Verification items for the finished model (mm, model axes). A direction names the side the tool comes from. Round coordinates to 2 decimals unless told otherwise and drop trailing zeros. Loops run counter-clockwise (first coordinate to the right, second up) from the corner with the lowest first, then second, coordinate; pieces in that order, holes last. Notation, with made-up numbers: M 42,67 L 83,67 A20 cw 83,85 Z; hole C 11,82.25 d10. An arc over 180 degrees is marked long. Write item = value, one per line. Start each with the question number.
from build123d import *

# Parameters (mm, degrees)
SKETCH1_W                  = 30
SKETCH1_H                  = 330
BOSS_EXTRUDE1_DEPTH        = 8.4
SKETCH2_R                  = 1
CUT_EXTRUDE1_DEPTH         = 332.467283453
LPATTERN1_COUNT            = 30
LPATTERN1_PITCH            = 8.5
LPATTERN2_COUNT            = 2
LPATTERN2_PITCH            = 22
LPATTERN2_COPY_1_SKETCH_R  = 1
LPATTERN2_COPY_1_DEPTH     = 332.467283453
LPATTERN2_COPY_2_SKETCH_R  = 1
LPATTERN2_COPY_2_DEPTH     = 332.467283453
LPATTERN2_COPY_3_SKETCH_R  = 1
LPATTERN2_COPY_3_DEPTH     = 332.467283453
LPATTERN2_COPY_4_SKETCH_R  = 1
LPATTERN2_COPY_4_DEPTH     = 332.467283453
LPATTERN2_COPY_5_SKETCH_R  = 1
LPATTERN2_COPY_5_DEPTH     = 332.467283453
LPATTERN2_COPY_6_SKETCH_R  = 1
LPATTERN2_COPY_6_DEPTH     = 332.467283453
LPATTERN2_COPY_7_SKETCH_R  = 1
LPATTERN2_COPY_7_DEPTH     = 332.467283453
LPATTERN2_COPY_8_SKETCH_R  = 1
LPATTERN2_COPY_8_DEPTH     = 332.467283453
LPATTERN2_COPY_9_SKETCH_R  = 1
LPATTERN2_COPY_9_DEPTH     = 332.467283453
LPATTERN2_COPY_10_SKETCH_R = 1
LPATTERN2_COPY_10_DEPTH    = 332.467283453
LPATTERN2_COPY_11_SKETCH_R = 1
LPATTERN2_COPY_11_DEPTH    = 332.467283453
LPATTERN2_COPY_12_SKETCH_R = 1
LPATTERN2_COPY_12_DEPTH    = 332.467283453
LPATTERN2_COPY_13_SKETCH_R = 1
LPATTERN2_COPY_13_DEPTH    = 332.467283453
LPATTERN2_COPY_14_SKETCH_R = 1
LPATTERN2_COPY_14_DEPTH    = 332.467283453
LPATTERN2_COPY_15_SKETCH_R = 1
LPATTERN2_COPY_15_DEPTH    = 332.467283453
LPATTERN2_COPY_16_SKETCH_R = 1
LPATTERN2_COPY_16_DEPTH    = 332.467283453
LPATTERN2_COPY_17_SKETCH_R = 1
LPATTERN2_COPY_17_DEPTH    = 332.467283453
LPATTERN2_COPY_18_SKETCH_R = 1
LPATTERN2_COPY_18_DEPTH    = 332.467283453
LPATTERN2_COPY_19_SKETCH_R = 1
LPATTERN2_COPY_19_DEPTH    = 332.467283453
LPATTERN2_COPY_20_SKETCH_R = 1
LPATTERN2_COPY_20_DEPTH    = 332.467283453
LPATTERN2_COPY_21_SKETCH_R = 1
LPATTERN2_COPY_21_DEPTH    = 332.467283453
LPATTERN2_COPY_22_SKETCH_R = 1
LPATTERN2_COPY_22_DEPTH    = 332.467283453
LPATTERN2_COPY_23_SKETCH_R = 1
LPATTERN2_COPY_23_DEPTH    = 332.467283453
LPATTERN2_COPY_24_SKETCH_R = 1
LPATTERN2_COPY_24_DEPTH    = 332.467283453
LPATTERN2_COPY_25_SKETCH_R = 1
LPATTERN2_COPY_25_DEPTH    = 332.467283453
LPATTERN2_COPY_26_SKETCH_R = 1
LPATTERN2_COPY_26_DEPTH    = 332.467283453
LPATTERN2_COPY_27_SKETCH_R = 1
LPATTERN2_COPY_27_DEPTH    = 332.467283453
LPATTERN2_COPY_28_SKETCH_R = 1
LPATTERN2_COPY_28_DEPTH    = 332.467283453
LPATTERN2_COPY_29_SKETCH_R = 1
LPATTERN2_COPY_29_DEPTH    = 332.467283453
SKETCH4_W                  = 24
SKETCH4_H                  = 65
CUT_EXTRUDE2_DEPTH         = 1.6
SKETCH6_W                  = 24
SKETCH6_H                  = 10
CUT_EXTRUDE3_DEPTH         = 1.6
SKETCH7_W                  = 30
SKETCH7_H                  = 8.4
BOSS_EXTRUDE2_DEPTH        = 2
SKETCH8_R                  = 2.5
CUT_EXTRUDE4_DEPTH         = 334.458483173


with BuildPart() as part:
    # Sketch1 → Boss-Extrude1 (new body)
    with BuildSketch(Plane.XY):
        with Locations((15, 165)):
            Rectangle(SKETCH1_W, SKETCH1_H)
    extrude(amount=BOSS_EXTRUDE1_DEPTH)

    # Sketch2 → Cut-Extrude1 (cut, through all)
    with BuildSketch(Plane.XY.offset(8.4)):
        with Locations((26, 4)):
            Circle(SKETCH2_R)
    cut_extrude1 = extrude(amount=-CUT_EXTRUDE1_DEPTH, mode=Mode.SUBTRACT)

    # LPattern1: Cut-Extrude1 ×30
    with Locations(*[(0, i * LPATTERN1_PITCH, 0) for i in range(1, LPATTERN1_COUNT)]):
        add(cut_extrude1, mode=Mode.SUBTRACT)

    # LPattern2: Cut-Extrude1 ×2
    with Locations(*[(-i * LPATTERN2_PITCH, 0, 0) for i in range(1, LPATTERN2_COUNT)]):
        add(cut_extrude1, mode=Mode.SUBTRACT)

    # LPattern2 copy 1 sketch → LPattern2 copy 1 (cut, through all)
    with BuildSketch(Plane(origin=(-22, 8.5, 8.4), x_dir=(1, 0, 0), z_dir=(0, 0, 1))):
        with Locations((26, 4)):
            Circle(LPATTERN2_COPY_1_SKETCH_R)
    extrude(amount=-LPATTERN2_COPY_1_DEPTH, mode=Mode.SUBTRACT)

    # LPattern2 copy 2 sketch → LPattern2 copy 2 (cut, through all)
    with BuildSketch(Plane(origin=(-22, 17, 8.4), x_dir=(1, 0, 0), z_dir=(0, 0, 1))):
        with Locations((26, 4)):
            Circle(LPATTERN2_COPY_2_SKETCH_R)
    extrude(amount=-LPATTERN2_COPY_2_DEPTH, mode=Mode.SUBTRACT)

    # LPattern2 copy 3 sketch → LPattern2 copy 3 (cut, through all)
    with BuildSketch(Plane(origin=(-22, 25.5, 8.4), x_dir=(1, 0, 0), z_dir=(0, 0, 1))):
        with Locations((26, 4)):
            Circle(LPATTERN2_COPY_3_SKETCH_R)
    extrude(amount=-LPATTERN2_COPY_3_DEPTH, mode=Mode.SUBTRACT)

    # LPattern2 copy 4 sketch → LPattern2 copy 4 (cut, through all)
    with BuildSketch(Plane(origin=(-22, 34, 8.4), x_dir=(1, 0, 0), z_dir=(0, 0, 1))):
        with Locations((26, 4)):
            Circle(LPATTERN2_COPY_4_SKETCH_R)
    extrude(amount=-LPATTERN2_COPY_4_DEPTH, mode=Mode.SUBTRACT)

    # LPattern2 copy 5 sketch → LPattern2 copy 5 (cut, through all)
    with BuildSketch(Plane(origin=(-22, 42.5, 8.4), x_dir=(1, 0, 0), z_dir=(0, 0, 1))):
        with Locations((26, 4)):
            Circle(LPATTERN2_COPY_5_SKETCH_R)
    extrude(amount=-LPATTERN2_COPY_5_DEPTH, mode=Mode.SUBTRACT)

    # LPattern2 copy 6 sketch → LPattern2 copy 6 (cut, through all)
    with BuildSketch(Plane(origin=(-22, 51, 8.4), x_dir=(1, 0, 0), z_dir=(0, 0, 1))):
        with Locations((26, 4)):
            Circle(LPATTERN2_COPY_6_SKETCH_R)
    extrude(amount=-LPATTERN2_COPY_6_DEPTH, mode=Mode.SUBTRACT)

    # LPattern2 copy 7 sketch → LPattern2 copy 7 (cut, through all)
    with BuildSketch(Plane(origin=(-22, 59.5, 8.4), x_dir=(1, 0, 0), z_dir=(0, 0, 1))):
        with Locations((26, 4)):
            Circle(LPATTERN2_COPY_7_SKETCH_R)
    extrude(amount=-LPATTERN2_COPY_7_DEPTH, mode=Mode.SUBTRACT)

    # LPattern2 copy 8 sketch → LPattern2 copy 8 (cut, through all)
    with BuildSketch(Plane(origin=(-22, 68, 8.4), x_dir=(1, 0, 0), z_dir=(0, 0, 1))):
        with Locations((26, 4)):
            Circle(LPATTERN2_COPY_8_SKETCH_R)
    extrude(amount=-LPATTERN2_COPY_8_DEPTH, mode=Mode.SUBTRACT)

    # LPattern2 copy 9 sketch → LPattern2 copy 9 (cut, through all)
    with BuildSketch(Plane(origin=(-22, 76.5, 8.4), x_dir=(1, 0, 0), z_dir=(0, 0, 1))):
        with Locations((26, 4)):
            Circle(LPATTERN2_COPY_9_SKETCH_R)
    extrude(amount=-LPATTERN2_COPY_9_DEPTH, mode=Mode.SUBTRACT)

    # LPattern2 copy 10 sketch → LPattern2 copy 10 (cut, through all)
    with BuildSketch(Plane(origin=(-22, 85, 8.4), x_dir=(1, 0, 0), z_dir=(0, 0, 1))):
        with Locations((26, 4)):
            Circle(LPATTERN2_COPY_10_SKETCH_R)
    extrude(amount=-LPATTERN2_COPY_10_DEPTH, mode=Mode.SUBTRACT)

    # LPattern2 copy 11 sketch → LPattern2 copy 11 (cut, through all)
    with BuildSketch(Plane(origin=(-22, 93.5, 8.4), x_dir=(1, 0, 0), z_dir=(0, 0, 1))):
        with Locations((26, 4)):
            Circle(LPATTERN2_COPY_11_SKETCH_R)
    extrude(amount=-LPATTERN2_COPY_11_DEPTH, mode=Mode.SUBTRACT)

    # LPattern2 copy 12 sketch → LPattern2 copy 12 (cut, through all)
    with BuildSketch(Plane(origin=(-22, 102, 8.4), x_dir=(1, 0, 0), z_dir=(0, 0, 1))):
        with Locations((26, 4)):
            Circle(LPATTERN2_COPY_12_SKETCH_R)
    extrude(amount=-LPATTERN2_COPY_12_DEPTH, mode=Mode.SUBTRACT)

    # LPattern2 copy 13 sketch → LPattern2 copy 13 (cut, through all)
    with BuildSketch(Plane(origin=(-22, 110.5, 8.4), x_dir=(1, 0, 0), z_dir=(0, 0, 1))):
        with Locations((26, 4)):
            Circle(LPATTERN2_COPY_13_SKETCH_R)
    extrude(amount=-LPATTERN2_COPY_13_DEPTH, mode=Mode.SUBTRACT)

    # LPattern2 copy 14 sketch → LPattern2 copy 14 (cut, through all)
    with BuildSketch(Plane(origin=(-22, 119, 8.4), x_dir=(1, 0, 0), z_dir=(0, 0, 1))):
        with Locations((26, 4)):
            Circle(LPATTERN2_COPY_14_SKETCH_R)
    extrude(amount=-LPATTERN2_COPY_14_DEPTH, mode=Mode.SUBTRACT)

    # LPattern2 copy 15 sketch → LPattern2 copy 15 (cut, through all)
    with BuildSketch(Plane(origin=(-22, 127.5, 8.4), x_dir=(1, 0, 0), z_dir=(0, 0, 1))):
        with Locations((26, 4)):
            Circle(LPATTERN2_COPY_15_SKETCH_R)
    extrude(amount=-LPATTERN2_COPY_15_DEPTH, mode=Mode.SUBTRACT)

    # LPattern2 copy 16 sketch → LPattern2 copy 16 (cut, through all)
    with BuildSketch(Plane(origin=(-22, 136, 8.4), x_dir=(1, 0, 0), z_dir=(0, 0, 1))):
        with Locations((26, 4)):
            Circle(LPATTERN2_COPY_16_SKETCH_R)
    extrude(amount=-LPATTERN2_COPY_16_DEPTH, mode=Mode.SUBTRACT)

    # LPattern2 copy 17 sketch → LPattern2 copy 17 (cut, through all)
    with BuildSketch(Plane(origin=(-22, 144.5, 8.4), x_dir=(1, 0, 0), z_dir=(0, 0, 1))):
        with Locations((26, 4)):
            Circle(LPATTERN2_COPY_17_SKETCH_R)
    extrude(amount=-LPATTERN2_COPY_17_DEPTH, mode=Mode.SUBTRACT)

    # LPattern2 copy 18 sketch → LPattern2 copy 18 (cut, through all)
    with BuildSketch(Plane(origin=(-22, 153, 8.4), x_dir=(1, 0, 0), z_dir=(0, 0, 1))):
        with Locations((26, 4)):
            Circle(LPATTERN2_COPY_18_SKETCH_R)
    extrude(amount=-LPATTERN2_COPY_18_DEPTH, mode=Mode.SUBTRACT)

    # LPattern2 copy 19 sketch → LPattern2 copy 19 (cut, through all)
    with BuildSketch(Plane(origin=(-22, 161.5, 8.4), x_dir=(1, 0, 0), z_dir=(0, 0, 1))):
        with Locations((26, 4)):
            Circle(LPATTERN2_COPY_19_SKETCH_R)
    extrude(amount=-LPATTERN2_COPY_19_DEPTH, mode=Mode.SUBTRACT)

    # LPattern2 copy 20 sketch → LPattern2 copy 20 (cut, through all)
    with BuildSketch(Plane(origin=(-22, 170, 8.4), x_dir=(1, 0, 0), z_dir=(0, 0, 1))):
        with Locations((26, 4)):
            Circle(LPATTERN2_COPY_20_SKETCH_R)
    extrude(amount=-LPATTERN2_COPY_20_DEPTH, mode=Mode.SUBTRACT)

    # LPattern2 copy 21 sketch → LPattern2 copy 21 (cut, through all)
    with BuildSketch(Plane(origin=(-22, 178.5, 8.4), x_dir=(1, 0, 0), z_dir=(0, 0, 1))):
        with Locations((26, 4)):
            Circle(LPATTERN2_COPY_21_SKETCH_R)
    extrude(amount=-LPATTERN2_COPY_21_DEPTH, mode=Mode.SUBTRACT)

    # LPattern2 copy 22 sketch → LPattern2 copy 22 (cut, through all)
    with BuildSketch(Plane(origin=(-22, 187, 8.4), x_dir=(1, 0, 0), z_dir=(0, 0, 1))):
        with Locations((26, 4)):
            Circle(LPATTERN2_COPY_22_SKETCH_R)
    extrude(amount=-LPATTERN2_COPY_22_DEPTH, mode=Mode.SUBTRACT)

    # LPattern2 copy 23 sketch → LPattern2 copy 23 (cut, through all)
    with BuildSketch(Plane(origin=(-22, 195.5, 8.4), x_dir=(1, 0, 0), z_dir=(0, 0, 1))):
        with Locations((26, 4)):
            Circle(LPATTERN2_COPY_23_SKETCH_R)
    extrude(amount=-LPATTERN2_COPY_23_DEPTH, mode=Mode.SUBTRACT)

    # LPattern2 copy 24 sketch → LPattern2 copy 24 (cut, through all)
    with BuildSketch(Plane(origin=(-22, 204, 8.4), x_dir=(1, 0, 0), z_dir=(0, 0, 1))):
        with Locations((26, 4)):
            Circle(LPATTERN2_COPY_24_SKETCH_R)
    extrude(amount=-LPATTERN2_COPY_24_DEPTH, mode=Mode.SUBTRACT)

    # LPattern2 copy 25 sketch → LPattern2 copy 25 (cut, through all)
    with BuildSketch(Plane(origin=(-22, 212.5, 8.4), x_dir=(1, 0, 0), z_dir=(0, 0, 1))):
        with Locations((26, 4)):
            Circle(LPATTERN2_COPY_25_SKETCH_R)
    extrude(amount=-LPATTERN2_COPY_25_DEPTH, mode=Mode.SUBTRACT)

    # LPattern2 copy 26 sketch → LPattern2 copy 26 (cut, through all)
    with BuildSketch(Plane(origin=(-22, 221, 8.4), x_dir=(1, 0, 0), z_dir=(0, 0, 1))):
        with Locations((26, 4)):
            Circle(LPATTERN2_COPY_26_SKETCH_R)
    extrude(amount=-LPATTERN2_COPY_26_DEPTH, mode=Mode.SUBTRACT)

    # LPattern2 copy 27 sketch → LPattern2 copy 27 (cut, through all)
    with BuildSketch(Plane(origin=(-22, 229.5, 8.4), x_dir=(1, 0, 0), z_dir=(0, 0, 1))):
        with Locations((26, 4)):
            Circle(LPATTERN2_COPY_27_SKETCH_R)
    extrude(amount=-LPATTERN2_COPY_27_DEPTH, mode=Mode.SUBTRACT)

    # LPattern2 copy 28 sketch → LPattern2 copy 28 (cut, through all)
    with BuildSketch(Plane(origin=(-22, 238, 8.4), x_dir=(1, 0, 0), z_dir=(0, 0, 1))):
        with Locations((26, 4)):
            Circle(LPATTERN2_COPY_28_SKETCH_R)
    extrude(amount=-LPATTERN2_COPY_28_DEPTH, mode=Mode.SUBTRACT)

    # LPattern2 copy 29 sketch → LPattern2 copy 29 (cut, through all)
    with BuildSketch(Plane(origin=(-22, 246.5, 8.4), x_dir=(1, 0, 0), z_dir=(0, 0, 1))):
        with Locations((26, 4)):
            Circle(LPATTERN2_COPY_29_SKETCH_R)
    extrude(amount=-LPATTERN2_COPY_29_DEPTH, mode=Mode.SUBTRACT)

    # Sketch4 → Cut-Extrude2 (cut)
    with BuildSketch(Plane.XY.offset(8.4)):
        with Locations((15, 297.5)):
            Rectangle(SKETCH4_W, SKETCH4_H)
    extrude(amount=-CUT_EXTRUDE2_DEPTH, mode=Mode.SUBTRACT)

    # Sketch6 → Cut-Extrude3 (cut)
    with BuildSketch(Plane.XY.offset(6.8)):
        with Locations((15, 325)):
            Rectangle(SKETCH6_W, SKETCH6_H)
    extrude(amount=-CUT_EXTRUDE3_DEPTH, mode=Mode.SUBTRACT)

    # Sketch7 → Boss-Extrude2 (add)
    with BuildSketch(Plane(origin=(0, 330, 0), x_dir=(1, 0, 0), z_dir=(0, 1, 0))):
        with Locations((15, -4.2)):
            Rectangle(SKETCH7_W, SKETCH7_H)
    extrude(amount=BOSS_EXTRUDE2_DEPTH)

    # Sketch8 → Cut-Extrude4 (cut, through all)
    with BuildSketch(Plane.XY.offset(8.4)):
        with Locations((10.5, 16)):
            Circle(SKETCH8_R)
        with Locations((19.5, 257)):
            Circle(SKETCH8_R)
        with Locations((19.5, 16)):
            Circle(SKETCH8_R)
        with Locations((10.5, 257)):
            Circle(SKETCH8_R)
    extrude(amount=-CUT_EXTRUDE4_DEPTH, mode=Mode.SUBTRACT)


solid = part.part
1. Mould release check, pull along X, two halves, no side actions. Record for faces 1 (the flat face through (15, 325, 5.2)), 2 (the flat face through (0, 164, 4)), 3 (the flat face through (15, 0, 4)): pulls with the +X half, pulls with the -X half, needs draft (parallel to the pull), parting line crosses it, or undercut.
2. Section check A-A, the plane y = 281.5. Enter the section's corners in (x, z), and give its area (3 significant figures).
3. Section check B-B, the plane z = 2.5. Give the number of separate pieces and of enclosed holes in the cut face, and give its area (3 significant figures).
4. Tool access check on faces 4 (the flat face through (15, 293, 6.8)), 5 (the flat face through (15, 127, 8.4)). Record the directions out of +Z, -Z, +X, -X, +Y, -Y that give a thin tool (end or side, any length) a straight path to the whole face; none if there is none.
5. Thickness scan on line 1 (Y direction, x = 10.5, z = 2); line 2 (X direction, y = 89, z = 6.75); line 3 (Y direction, x = 10.5, z = 6). Record the ranges inside material, lowest first.
Computed values:
q1.face_1 = undercut
q1.face_2 = pulls with the -X half
q1.face_3 = needs draft
q2.outline = M 0,0 L 30,0 L 30,8.4 L 27,8.4 L 27,6.8 L 3,6.8 L 3,8.4 L 0,8.4 Z
q2.area = 214 mm2
q3.separate_pieces = 1
q3.enclosed_holes = 64
q3.area = 9,690 mm2
q4.face_4 = +Z
q4.face_5 = +Z, +X, -X, +Y, -Y
q5.line_1 = 0 to 13.5, 18.5 to 254.5, 259.5 to 332
q5.line_2 = 0 to 3, 5 to 25, 27 to 30
q5.line_3 = 0 to 13.5, 18.5 to 254.5, 259.5 to 320, 330 to 332
